Input: part model. Units: mm. Frame: model coordinates. Face numbers are marked on the shaded views. A direction names the side the tool comes from. Round coordinates to 2 decimals unless told otherwise and drop trailing zeros. Loops run counter-clockwise (first coordinate to the right, second up) from the corner with the lowest first, then second, coordinate; pieces in that order, holes last. Notation, with made-up numbers: (2.25, 84.5) -> (30.25, 84.5) arc R9 cw to (30.25, 91.5) -> close; hole circle Ø11 at (5.25, -25.5). An arc over 180 degrees is marked (long way). Answer in a Markdown table with one row per item. Add a question column.
Q1. Section C-C, the plane y = -2.5. Output: boundary loops of the cut face in (x, z).
Q2. Pin query (flat end, axial travel): pin 1 (5.5 mm diameter, centred on x = 11.5, z = 9.5, fed in from +Y); pin 2 (3 mm diameter, centred on y = -7, z = -0.5, fed in from +X). Return the tip coordinate at first contact, or that it passes through.
Q3. Reachability of the marked faces 3, 4, 5 and 6 from +Z, -Z, +X, -X, +Y, -Y: full face, straight path, thin tool, end or side. Return the list, or none.
Q4. Section D-D, the plane z = 5. Output: boundary loops of the cut face in (x, y).
Q5. Section A-A, the plane x = -4.5. Output: boundary loops of the cut face in (y, z).
Q6. Mould query, pull axis X, two halves, no side actions, for the marked faces 1 and 2. Classes: pulls with the +X half, pulls with the -X half, needs draft (parallel to the pull), parting line crosses it, or undercut.
Q7. Section B-B, the plane y = 0.75. Output: boundary loops of the cut face in (x, z).
Q8. Ray query, L1, parallel to Y at x = -4.5, z = -11.5; L2, parallel to Y at x = -5.5, z = -1.5; L3, parallel to X at y = -17.5, z = -10.5. Return the intervals inside material, ascending. Write a range as from..to.
Autodesk Inventor part; units mm, degrees
ref_plane "YZ Plane" through (0, 0, 0) normal (1, 0, 0) x (0, 1, 0)
ref_plane "XZ Plane" through (0, 0, 0) normal (0, 1, 0) x (-1, 0, 0)
ref_plane "XY Plane" through (0, 0, 0) normal (0, 0, 1) x (1, 0, 0)
sketch "Sketch1" plane through (0, 0, 0) normal (0, 1, 0) x (-1, 0, 0)
  line L0 (7.1862, 13.3676) -> (-7.8138, 13.3676)
  line L1 (-7.8138, 13.3676) -> (-7.8138, -19.1776)
  line L2 (-7.8138, -19.1776) -> (7.1862, -19.1776)
  line L3 (7.1862, -19.1776) -> (7.1862, 13.3676)
  point P0 (0, 0)
  dimension "d0" = 15
extrude "Extrusion1" add sketch "Sketch1" along normal blind 3
sketch "Sketch2" plane through (0, 3, 0) normal (0, 1, 0) x (1, 0, 0)
  line L0 (0.84, -11.5857) -> (6.3178, -11.5857)
  line L1 (6.3178, -11.5857) -> (6.3178, -6.6455)
  line L2 (6.3178, -6.6455) -> (0.84, -6.6455)
  line L3 (0.84, -6.6455) -> (0.84, -11.5857)
  point P0 (0, 0)
extrude "Extrusion2" cut sketch "Sketch2" against normal blind 4.5
sketch "Sketch3" plane through (0, 3, 0) normal (0, 1, 0) x (1, 0, 0)
  line L0 (-6.4027, 18.2927) -> (-3.3498, 18.2927)
  line L1 (-3.3498, 18.2927) -> (-3.3498, 8.0094)
  line L2 (-3.3498, 8.0094) -> (-6.4027, 8.0094)
  line L3 (-6.4027, 8.0094) -> (-6.4027, 18.2927)
  point P0 (0, 0)
extrude "Extrusion3" add sketch "Sketch3" along normal blind 1.5
sketch "Sketch4" plane through (-7.1862, 0, 13.3676) normal (0, 0, 1) x (1, 0, 0)
  line L0 (0, 3) -> (15, 3)
  line L1 (0, 3) -> (15, 3)
  line L2 (15, 3) -> (15, -19.0502)
  line L3 (15, -19.0502) -> (0, -19.0502)
  line L4 (0, -19.0502) -> (0, 3)
  point P0 (7.1862, 0)
extrude "Extrusion4" add sketch "Sketch4" along normal blind 1.5
sketch "Sketch5" plane through (-7.1862, 0, 13.3676) normal (0, 0, -1) x (-1, 0, 0)
  line L0 (-15, -19.0502) -> (-15, 0)
  line L1 (0, 0) -> (0, -19.0502)
  line L2 (-15, -6.2009) -> (0, -6.2009)
  line L3 (0, -6.2009) -> (0, -4.8004)
  line L4 (0, -4.8004) -> (-15, -4.8004)
  line L5 (-15, -4.8004) -> (-15, -6.2009)
  point P0 (-7.1862, 0)
extrude "Extrusion5" add sketch "Sketch5" along normal blind 32.5
sketch "Sketch6" plane through (7.8138, 0, -19.1776) normal (0, 0, -1) x (-1, 0, 0)
  line L0 (0, 0) -> (0, 3)
  line L1 (15, -6.2009) -> (15, -19.0502)
  line L2 (0, 3) -> (15, 3)
  line L3 (15, 3) -> (15, -19.0502)
  line L4 (15, -19.0502) -> (0, -19.0502)
  line L5 (0, -19.0502) -> (0, 3)
  point P0 (7.8138, 0)
extrude "Extrusion6" add sketch "Sketch6" along normal blind 1.5
sketch "Sketch7" plane through (-7.1862, -19.0502, -19.1776) normal (0, -1, 0) x (1, 0, 0)
  line L0 (15, -1.5) -> (15, 34.0452)
  line L1 (15, -1.5) -> (0, -1.5)
  line L2 (0, -1.5) -> (0, 34.0452)
  line L3 (0, 34.0452) -> (15, 34.0452)
  line L4 (15, 34.0452) -> (15, -1.5)
  point P0 (7.1862, 19.1776)
extrude "Extrusion7" add sketch "Sketch7" along normal blind 1.5
sketch "Sketch8" plane through (0, 3, 0) normal (0, 1, 0) x (1, 0, 0)
  point P0 (0, 0)
sketch "Sketch10" plane through (7.8138, 3, 14.8676) normal (1, 0, 0) x (0, 0, -1)
  line L0 (0, 0) -> (35.5452, 0)
  line L1 (35.5452, 0) -> (35.5452, -23.5502)
  line L2 (0, 0) -> (35.5452, 0)
  line L3 (35.5452, 0) -> (35.5452, -23.5502)
  line L4 (35.5452, -23.5502) -> (0, -23.5502)
  line L5 (0, -23.5502) -> (0, 0)
  point P0 (14.8676, -3)
extrude "Extrusion9" add sketch "Sketch10" along normal blind 1.5
sketch "Sketch11" plane through (9.3138, 3, 14.8676) normal (1, 0, 0) x (0, 0, -1)
  point P0 (14.8676, -3)
sketch "Sketch12" plane through (9.3138, 3, 14.8676) normal (1, 0, 0) x (0, 0, -1)
  line L0 (1.5, -7.8004) -> (34, -7.8004)
  line L1 (2.6857, -1.2569) -> (7.8665, -1.2569)
  line L2 (7.8665, -1.2569) -> (7.8665, -7.8004)
  line L3 (7.8665, -7.8004) -> (2.6857, -7.8004)
  line L4 (2.6857, -7.8004) -> (2.6857, -1.2569)
  point P0 (14.8676, -3)
  point P1 (2.6857, -7.8004)
extrude "Extrusion10" cut sketch "Sketch12" against normal blind 1.5
sketch "Sketch13" plane through (-7.1862, -19.0502, -19.1776) normal (0, 1, 0) x (1, 0, 0)
  line L0 (11.8023, -6.3584) -> (1.3351, -6.3584)
  line L1 (1.3351, -6.3584) -> (1.3351, -31.4677)
  line L2 (1.3351, -31.4677) -> (11.8023, -31.4677)
  line L3 (11.8023, -31.4677) -> (11.8023, -6.3584)
  point P0 (7.1862, -19.1776)
extrude "Extrusion11" add sketch "Sketch13" along normal blind 1
sketch "Sketch14" plane through (-7.1862, -18.0502, -19.1776) normal (0, 1, 0) x (1, 0, 0)
  line L0 (10.9591, -8.0288) -> (2.1896, -8.0288)
  line L1 (2.1896, -8.0288) -> (2.1896, -30.8703)
  line L2 (2.1896, -30.8703) -> (10.9591, -30.8703)
  line L3 (10.9591, -30.8703) -> (10.9591, -8.0288)
  point P0 (7.1862, -19.1776)
extrude "Extrusion12" add sketch "Sketch14" along normal blind 1
sketch "Sketch15" plane through (-7.1862, -4.8004, 13.3676) normal (0, 1, 0) x (1, 0, 0)
  line L0 (12.3187, 15.0671) -> (8.4438, 15.0671)
  line L1 (8.4438, 15.0671) -> (8.4438, 7.8611)
  line L2 (8.4438, 7.8611) -> (12.3187, 7.8611)
  line L3 (12.3187, 7.8611) -> (12.3187, 15.0671)
  point P0 (7.1862, 13.3676)
extrude "Extrusion13" add sketch "Sketch15" along normal blind 1
sketch "Sketch17" plane through (-7.1862, -17.0502, -19.1776) normal (0, 1, 0) x (1, 0, 0)
  line L0 (8.3336, -13.5877) -> (3.2144, -13.5877)
  line L1 (3.2144, -13.5877) -> (3.2144, -29.2984)
  line L2 (3.2144, -29.2984) -> (8.3336, -29.2984)
  line L3 (8.3336, -29.2984) -> (8.3336, -13.5877)
  point P0 (7.1862, -19.1776)
extrude "Extrusion15" add sketch "Sketch17" along normal blind 1
sketch "Sketch19" plane through (7.8138, 3, 14.8676) normal (1, 0, 0) x (0, 0, -1)
  line L0 (2.6857, -1.2569) -> (7.8665, -1.2569)
  line L1 (7.8665, -1.2569) -> (7.8665, -7.8004)
  line L2 (2.6857, -1.2569) -> (7.8665, -1.2569)
  line L3 (7.8665, -1.2569) -> (7.8665, -3)
  line L4 (7.8665, -3) -> (2.6857, -3)
  line L5 (2.6857, -3) -> (2.6857, -1.2569)
  point P0 (14.8676, -3)
extrude "Extrusion16" add sketch "Sketch19" along normal blind 7
sketch "Sketch20" plane through (-7.1862, -4.8004, 13.3676) normal (0, 1, 0) x (1, 0, 0)
  point P0 (7.1862, 13.3676)
sketch "Sketch21" plane through (-7.1862, -4.8004, 13.3676) normal (0, 1, 0) x (1, 0, 0)
  point P0 (7.1862, 13.3676)
sketch "Sketch22" plane through (-7.1862, -4.8004, 13.3676) normal (0, 1, 0) x (1, 0, 0)
  point P0 (7.1862, 13.3676)
sketch "Sketch23" plane through (-7.1862, -4.8004, 13.3676) normal (0, 1, 0) x (1, 0, 0)
  circle A0 centre (11.5182, 22.6981) radius 2.5447
  point P0 (7.1862, 13.3676)
extrude "Extrusion17" cut sketch "Sketch23" against normal blind 1.5
sketch "Sketch24" plane through (-7.1862, -4.8004, 13.3676) normal (0, 1, 0) x (1, 0, 0)
  point P0 (7.1862, 13.3676)
sketch "Sketch25" plane through (-7.1862, -4.8004, 13.3676) normal (0, 1, 0) x (1, 0, 0)
  point P0 (7.1862, 13.3676)
sketch "Sketch26" plane through (-7.1862, -4.8004, 13.3676) normal (0, 1, 0) x (1, 0, 0)
  point P0 (7.1862, 13.3676)
sketch "Sketch27" plane through (-7.1862, -4.8004, 13.3676) normal (0, 1, 0) x (1, 0, 0)
  line L0 (10.9591, 1.6749) -> (10.9591, 24.5164)
  circle A0 centre (10.9591, 4.3668) radius 1.0997
  point P0 (7.1862, 13.3676)
extrude "Extrusion18" cut sketch "Sketch27" against normal blind 1.5
sketch "Sketch28" plane through (0, 4.5, 0) normal (0, 1, 0) x (1, 0, 0)
  point P0 (0, 0)
properties part number "Atas"
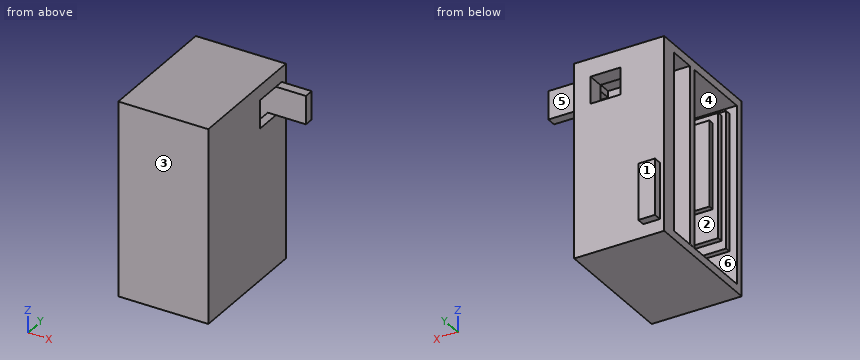
Answer block:
| question | item | result |
|---|---|---|
| 1 | outline | (-7.19, -20.68) -> (9.31, -20.68) -> (9.31, 7) -> (7.81, 7) -> (7.81, -19.18) -> (-7.19, -19.18) -> close; (-7.19, 13.37) -> (7.81, 13.37) -> (7.81, 12.18) -> (9.31, 12.18) -> (9.31, 14.87) -> (-7.19, 14.87) -> close |
| 2 | pin 1 | y = 3 |
| 2 | pin 2 | x = 9.31 |
| 3 | face 3 | +Z, -Z, +X, -X, -Y |
| 3 | face 4 | -X |
| 3 | face 5 | +Z, -Z, +X, +Y |
| 3 | face 6 | none |
| 4 | outline | (-7.19, -20.55) -> (9.31, -20.55) -> (9.31, 3) -> (-7.19, 3) -> (-7.19, 0) -> (7.81, 0) -> (7.81, -4.8) -> (5.13, -4.8) -> (5.13, -3.8) -> (1.26, -3.8) -> (1.26, -4.8) -> (-7.19, -4.8) -> (-7.19, -6.2) -> (7.81, -6.2) -> (7.81, -19.05) -> (4.62, -19.05) -> (4.62, -18.05) -> (3.77, -18.05) -> (3.77, -17.05) -> (1.15, -17.05) -> (1.15, -16.05) -> (-3.97, -16.05) -> (-3.97, -17.05) -> (-5, -17.05) -> (-5, -18.05) -> (-5.85, -18.05) -> (-5.85, -19.05) -> (-7.19, -19.05) -> close |
| 5 | outline | (-20.55, -20.68) -> (3, -20.68) -> (3, -18.29) -> (4.5, -18.29) -> (4.5, -8.01) -> (3, -8.01) -> (3, 14.87) -> (-20.55, 14.87) -> close; hole (-19.05, -19.18) -> (0, -19.18) -> (0, 13.37) -> (-4.8, 13.37) -> (-4.8, -19.13) -> (-6.2, -19.13) -> (-6.2, 13.37) -> (-19.05, 13.37) -> (-19.05, 12.29) -> (-18.05, 12.29) -> (-18.05, 11.69) -> (-17.05, 11.69) -> (-17.05, -11.15) -> (-18.05, -11.15) -> (-18.05, -12.82) -> (-19.05, -12.82) -> close |
| 6 | face 1 | needs draft |
| 6 | face 2 | undercut |
| 7 | outline | (-7.19, -20.68) -> (9.31, -20.68) -> (9.31, 7) -> (14.81, 7) -> (14.81, 12.18) -> (9.31, 12.18) -> (9.31, 14.87) -> (-7.19, 14.87) -> close; hole (0.84, 6.65) -> (6.32, 6.65) -> (6.32, 11.59) -> (0.84, 11.59) -> close |
| 8 | L1 | -20.55..-18.05, -6.2..-4.8, 0..4.5 |
| 8 | L2 | -20.55..-18.05, -6.2..-4.8, 0..3 |
| 8 | L3 | -5..3.77, 7.81..9.31 |
